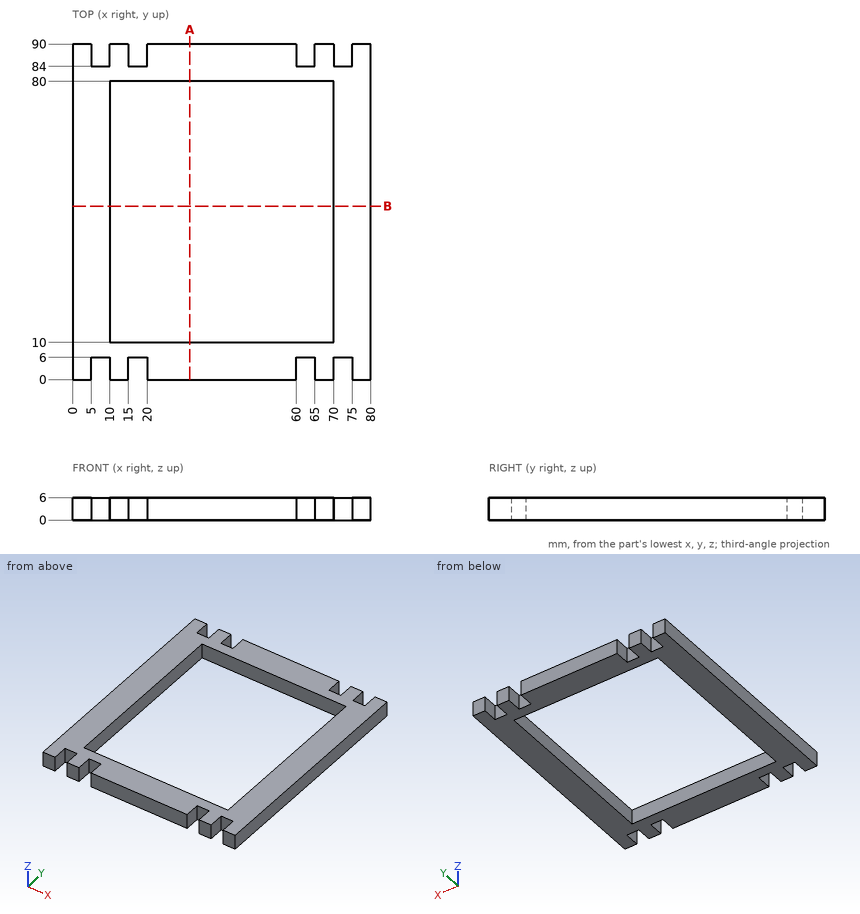
The drawing under review shows one solid part. Ordinate dimensions are in mm from its lowest x, y, z. Give positions to 0.01 mm unless a question says otherwise; leave off trailing zeros. Order: outer loops, then holes, each group sorted by start corner. A loop starts at its lowest first (then second) coordinate and runs counter-clockwise, first axis right, second up. Notation, with made-up numbers: (-9.5, 53.5) - (6.5, 53.5) arc R9 ccw to (6.5, 64.5) - close; hole circle Ø1 at (-32, 41.25). An arc over 180 degrees is marked (long way). Answer as a JSON object with one key per item and string values. Group by question number.
Item 1: Wall thickness on line 1 along X through (y, z) = (37, 3.65); line 2 along Y through (x, z) = (60.5, 5.15); line 3 along Y through (x, z) = (68, 3.9): over which ranges is each line inside the solid? List them lowest first.
Item 2: Clearance check with flat-ended pins moving along their axes: pin 1 Ø2.5 at (x, z) = (73.5, 3.5) entering from +Y; pin 2 Ø1.5 at (x, z) = (8, 2.5) entering from -Y. State where each tip first meets the part, or that it passes through.
Item 3: Take a section at B-B on y = 46.5. Give the boundary of the cut face in (x, z).
Item 4: Take a section at A-A on x = 31.5. Give the boundary of the cut face in (y, z).
Reported:
{
 "1": {"line 1": "0 to 10, 70 to 80", "line 2": "6 to 10, 80 to 84", "line 3": "0 to 10, 80 to 90"},
 "2": {"pin 1": "y = 84", "pin 2": "y = 6"},
 "3": {"outline": "(0, 0) - (10, 0) - (10, 6) - (0, 6) - close; (70, 0) - (80, 0) - (80, 6) - (70, 6) - close"},
 "4": {"outline": "(0, 0) - (10, 0) - (10, 6) - (0, 6) - close; (80, 0) - (90, 0) - (90, 6) - (80, 6) - close"}
}
